```python
from build123d import *

# Parameters (mm, degrees)
F0_W      = 228.6
F0_H      = 228.6
F1_DEPTH  = 609.6
F3_SIZE   = 40
F4_R      = 85
F5_DEPTH  = 25
F6_R      = 70
F7_DEPTH  = 46
F9_DEPTH  = 70
F10_W     = 32
F10_H     = 45.417998
F11_DEPTH = 252
F12_SIZE  = 20
F14_D     = 12
F14_DEPTH = 40


with BuildPart() as f1:
    # F0 (on Front) → F1 (new body)
    with BuildSketch(Plane.XZ):
        Rectangle(F0_W, F0_H)
    extrude(amount=F1_DEPTH)

    # F3
    f3_edges = [f1.edges().sort_by_distance(p)[0] for p in [
        (114.3, -304.8, 114.3),
        (-114.3, -304.8, 114.3),
        (-114.3, -304.8, -114.3),
        (114.3, -304.8, -114.3),
    ]]
    chamfer(f3_edges, length=F3_SIZE)

    # F4 (on Front) → F5 (join)
    with BuildSketch(Plane.XZ):
        Circle(F4_R)
    extrude(amount=-F5_DEPTH)

    # F6 (on face) → F7 (join)
    with BuildSketch(Plane(origin=(0, 25, 0), x_dir=(-1, 0, 0), z_dir=(0, 1, 0))):
        Circle(F6_R)
    extrude(amount=F7_DEPTH)

    # F8 (on face) → F9 (join)
    with BuildSketch(Plane(origin=(0, 71, 0), x_dir=(-1, 0, 0), z_dir=(0, 1, 0))):
        Polygon((-32, 95), (-72, 95), (-72, -95), (-32, -95), (-32, 0), align=None)
        Polygon((0, 95), (-32, 95), (-32, 0), (-32, -95), (0, -95), (0, 0), align=None)
        Polygon((36, 95), (0, 95), (0, 0), (0, -95), (36, -95), align=None)
    extrude(amount=F9_DEPTH)

    # F10 (on face) → F11 (cut)
    with BuildSketch(Plane(origin=(0, 0, -95), x_dir=(1, 0, 0), z_dir=(0, 0, -1))):
        with Locations((16, -127.708999)):
            Rectangle(F10_W, F10_H)
    extrude(amount=-F11_DEPTH, mode=Mode.SUBTRACT)

    # F12
    f12_edges = [f1.edges().sort_by_distance(p)[0] for p in [
        (72, 106, -95),
        (72, 106, 95),
    ]]
    chamfer(f12_edges, length=F12_SIZE)

    # F14
    with Locations(Plane(origin=(-36, 0, 0), x_dir=(0, -1, 0), z_dir=(-1, 0, 0))):
        with Locations((-128.494948, 80), (-128.494948, 40), (-128.494948, 0), (-128.494948, -40), (-128.494948, -80)):
            Hole(F14_D / 2, depth=F14_DEPTH)


solid = f1.part
```
Can you work these out from the model? Positions are in its coordinate system, mm. A direction names the side the tool comes from. Coordinates: 2 decimals unless noted, no trailing zeros. Loops run counter-clockwise (first coordinate to the right, second up) from the corner with the lowest first, then second, coordinate; pieces in that order, holes last.
1) I need wall thicknesses on probe 1 along Y at (x, z) = (62, -47.5); probe 2 along Y at (x, z) = (-68.5, 80.5); probe 3 along Y at (x, z) = (-69.5, -10). Which ranges of each line are inside material? Lowest first, please.
2) Imagine slicing it at C-C on y = 17. List the corners of the cut face in (x, z) for me, plus the area to 3 significant figures.
3) For pin 1 (21 mm diameter, centred on y = 91.5, z = -33.5, fed in from +X); pin 2 (11 mm diameter, centred on y = 128.49, z = 0, fed in from -X); pin 3 (3 mm diameter, centred on x = 0, y = 53.5, fed in from -Z), each with a flat end and sliding along its axis, tell me the tip position at first contact or that it passes through.
4) Imagine slicing it at A-A on y = -456.5. List the corners of the cut face in (x, z) for me, plus the area to 3 significant figures.
5) Which directions (+Z, -Z, +X, -X, +Y, -Y) give clear straight access to the entire face, cutting with the end or side of a thin tool? Please do faces 4 (the flat face through (12, 25, 70)), 5 (the flat face through (-49, 71, 1)), 6 (the flat face through (62, 106, 85)), 7 (the flat face through (7, 98, 95)).
6) Thinking about a two-plate mould opening in Y: for faces 1 (the flat face through (-1, -301, -114.3)), 2 (the flat face through (52, 141, 1)), 3 (the cylindrical face through (55.55, 47.678, -42.594)), which applies, pulls with the +Y half, pulls with the -Y half, needs draft (parallel to the pull), parting line crosses it, or undercut?
7) Imagine slicing it at B-B on x = 60. List the corners of the cut face in (y, z) for me, plus the area to 3 significant figures.
Completed:
1. probe 1: y = -609.6 to 25, 71 to 141
1. probe 2: y = -609.6 to 0
1. probe 3: y = -609.6 to 25
2. outline: circle Ø170 at (0, 0)
2. area: 22,700 mm2
3. pin 1: stops at x = 72
3. pin 2: stops at x = 32
3. pin 3: stops at z = -70
4. outline: (-114.3, -74.3) - (-74.3, -114.3) - (74.3, -114.3) - (114.3, -74.3) - (114.3, 74.3) - (74.3, 114.3) - (-74.3, 114.3) - (-114.3, 74.3) - close
4. area: 49,100 mm2
5. face 4: none
5. face 5: +Z, -Z, -X, +Y
5. face 6: +Z, +X, +Y
5. face 7: +Z, +X, -X, +Y
6. face 1: needs draft
6. face 2: pulls with the +Y half
6. face 3: undercut
7. outline: (-609.6, -114.3) - (0, -114.3) - (0, -60.21) - (25, -60.21) - (25, -36.06) - (71, -36.06) - (71, -87) - (141, -87) - (141, 87) - (71, 87) - (71, 36.06) - (25, 36.06) - (25, 60.21) - (0, 60.21) - (0, 114.3) - (-609.6, 114.3) - close
7. area: 158,000 mm2
